from build123d import *

# Parameters (mm, degrees)
F1_DEPTH       = 76.2
F3_D           = 15.24
F3_CBORE_D     = 40.64
F3_CBORE_DEPTH = 10.16
F5_DEPTH       = 76.2
F6_R           = 10.16
F7_DEPTH       = 76.2
F9_DEPTH       = 27.94
F10_R          = 10.16


with BuildPart() as f1:
    # F0 (on Right) → F1 (new body)
    with BuildSketch(Plane.YZ):
        Polygon((0, 35.56), (0, 0), (111.76, 0), (147.32, 35.56), (147.32, 71.12), (111.76, 71.12), (76.2, 35.56), align=None)
    extrude(amount=F1_DEPTH)

    # F3 (through all)
    with Locations(Plane.XY.offset(35.56)):
        with Locations((38.1, 38.1)):
            CounterBoreHole(F3_D / 2, F3_CBORE_D / 2, F3_CBORE_DEPTH)

    # F4 (on face) → F5 (cut)
    with BuildSketch(Plane.XZ):
        Polygon((40.64, 35.56), (38.1, 35.56), (35.56, 35.56), (35.56, 25.4), (40.64, 25.4), align=None)
    extrude(amount=-F5_DEPTH, mode=Mode.SUBTRACT)

    # F6 (on face) → F7 (cut)
    with BuildSketch(Plane.YZ.offset(76.2)):
        with Locations((93.98, 20.32)):
            Circle(F6_R)
    extrude(amount=-F7_DEPTH, mode=Mode.SUBTRACT)

    # F8 (on face) → F9 (cut)
    with BuildSketch(Plane.XY.offset(71.12)):
        with BuildLine():
            Line((60.96, 133.35), (15.24, 133.35))
            ThreePointArc((15.24, 133.35), (11.43, 129.54), (15.24, 125.73))
            Line((15.24, 125.73), (60.96, 125.73))
            ThreePointArc((60.96, 125.73), (64.77, 129.54), (60.96, 133.35))
        make_face()
    extrude(amount=-F9_DEPTH, mode=Mode.SUBTRACT)

    # F10
    f10_edges = [f1.edges().sort_by_distance(p)[0] for p in [
        (0, 0, 17.78),
        (76.2, 0, 17.78),
    ]]
    fillet(f10_edges, radius=F10_R)


solid = f1.part
Input: part model. Units: mm. Frame: model coordinates. A direction names the side the tool comes from. Round coordinates to 2 decimals unless told otherwise and drop trailing zeros. Order: outer loops, then holes, each group sorted by start corner. A loop starts at its lowest first (then second) coordinate and runs counter-clockwise, first axis right, second up. Notation, with made-up numbers: (86.25, 60) - (113.25, 60) arc R28 cw to (113.25, 83) - close; hole circle Ø4 at (13, 2). An arc over 180 degrees is marked (long way). Use a Markdown table: item, result.
1. Material intervals for probe 1 along Y at (x, z) = (38.1, 12); probe 2 along Y at (x, z) = (38.1, 11.25); probe 3 along X at (y, z) = (38, 16), sorted ascending.
Evaluation:
| item | result |
|---|---|
| probe 1 | 0 to 30.48, 45.72 to 88.15, 99.81 to 123.76 |
| probe 2 | 0 to 30.48, 45.72 to 89.4, 98.56 to 123.01 |
| probe 3 | 0 to 30.48, 45.72 to 76.2 |
2. Access query for faces 1 (the face through (38, 147.32, 53)), 2 (the face through (35.56, 67, 31)), 3 (the face through (58.416, 37.689, 30.551)), 4 (the face through (14, 39, 35.56)). Directions: +Z, -Z, +X, -X, +Y, -Y. A direction counts if a zero-diameter tool reaches every point of the face in a straight line with its end or side. Return the directions, or none.
Evaluation:
| item | result |
|---|---|
| face 1 | +Z, -Z, +X, -X, +Y |
| face 2 | +Z, -Y |
| face 3 | +Z |
| face 4 | +Z, +X, -X, -Y |
3. First-contact query: pin 1 (10 mm diameter, centred on x = 60.5, z = 25.5, fed in from +Y); pin 2 (4 mm diameter, centred on x = 32.5, y = 129, fed in from +Z); pin 3 (8.5 mm diameter, centred on x = 46.5, z = 52, fed in from -Y). Flat tips, straight axial feed; report the tip coordinate or a pass-through.
Evaluation:
| item | result |
|---|---|
| pin 1 | y = 142.26 |
| pin 2 | z = 43.18 |
| pin 3 | y = 88.39 |
4. Section A-A on x = 38.1. Return the cut outline in (y, z).
Evaluation:
| item | result |
|---|---|
| outline | (0, 0) - (30.48, 0) - (30.48, 25.4) - (0, 25.4) - close; (45.72, 0) - (111.76, 0) - (147.32, 35.56) - (147.32, 71.12) - (133.35, 71.12) - (133.35, 43.18) - (125.73, 43.18) - (125.73, 71.12) - (111.76, 71.12) - (76.2, 35.56) - (76.2, 25.4) - (45.72, 25.4) - close; hole circle Ø20.32 at (93.98, 20.32) |
5. Section C-C on z = 20.32. Return the cut outline in (x, y).
Evaluation:
| item | result |
|---|---|
| outline | (0, 10.16) arc R10.16 ccw to (10.16, 0) - (66.04, 0) arc R10.16 ccw to (76.2, 10.16) - (76.2, 83.82) - (0, 83.82) - close; (0, 104.14) - (76.2, 104.14) - (76.2, 132.08) - (0, 132.08) - close; hole circle Ø15.24 at (38.1, 38.1) |
6. Section D-D on z = 60.5. Return the cut outline in (x, y), then the cut area to 3 significant figures.
Evaluation:
| item | result |
|---|---|
| outline | (0, 101.14) - (76.2, 101.14) - (76.2, 147.32) - (0, 147.32) - close; hole (15.24, 125.73) - (60.96, 125.73) arc R3.81 ccw to (60.96, 133.35) - (15.24, 133.35) arc R3.81 ccw to start |
| area | 3,120 mm^2 |
7. Section B-B on y = 93.98. Return the cut outline in (x, z).
Evaluation:
| item | result |
|---|---|
| outline | (0, 0) - (76.2, 0) - (76.2, 10.16) - (0, 10.16) - close; (0, 30.48) - (76.2, 30.48) - (76.2, 53.34) - (0, 53.34) - close |
8. Mould query, pull axis X, two halves, no side actions, for faces 5 (the face through (37.57, 129.29, 17.53)), 6 (the face through (34.004, 44.525, 12.522)), 7 (the face through (3.055, 2.897, 17.531)). Classes: +X half, -X half, draft (parallel to the pull), parting line (faces both ways), or undercut.
Evaluation:
| item | result |
|---|---|
| face 5 | draft |
| face 6 | undercut |
| face 7 | -X half |
